Here's how the part is built. I have some questions about the finished solid (model axes, mm). A direction names the side the tool comes from. Round coordinates to 2 decimals unless told otherwise and drop trailing zeros. Loops run counter-clockwise (first coordinate to the right, second up) from the corner with the lowest first, then second, coordinate; pieces in that order, holes last. Notation, with made-up numbers: M 75,-8 L 130,-8 A8 ccw 130,1 Z; hole C 1,-13.75 d5. An arc over 180 degrees is marked long. Answer as CSV lines item,"result".
```python
from build123d import *

# Parameters (mm, degrees)
F0_W      = 45
F0_H      = 49
F1_DEPTH  = 80
F3_DEPTH  = 35
F4_W      = 72
F4_H      = 41
F5_DEPTH  = 55
F6_W      = 72
F6_H      = 23
F7_DEPTH  = 15
F9_W      = 80
F9_H      = 45
F9_R      = 8
F10_DEPTH = 14
F11_R     = 5
F13_DEPTH = 80


with BuildPart() as f1:
    # F0 (on Right) → F1 (new body)
    with BuildSketch(Plane.YZ):
        with Locations((22.5, -24.5)):
            Rectangle(F0_W, F0_H)
        Polygon((50, 86.6025403784), (0, 0), (45, 0), (95, 86.6025403784), align=None)
    extrude(amount=F1_DEPTH)

    # F2 (on face) → F3 (cut)
    with BuildSketch(Plane(origin=(0, 33.75, -19.4855715851), x_dir=(-1, 0, 0), z_dir=(0, 0.8660254038, -0.5))):
        Polygon((-76, 22.5), (-4, 22.5), (-4, 117.5), (-4, 122.5), (-76, 122.5), (-76, 117.5), align=None)
    extrude(amount=-F3_DEPTH, mode=Mode.SUBTRACT)

    # F4 (on face) → F5 (cut)
    with BuildSketch(Plane(origin=(0, 0, -49), x_dir=(1, 0, 0), z_dir=(0, 0, -1))):
        with Locations((40, -24.5)):
            Rectangle(F4_W, F4_H)
    extrude(amount=-F5_DEPTH, mode=Mode.SUBTRACT)

    # F6 (on face) → F7 (cut)
    with BuildSketch(Plane(origin=(0, 11.25, 19.4855715851), x_dir=(1, 0, 0), z_dir=(0, 0.5, 0.8660254038))):
        with Locations((40, 15.4711431703)):
            Rectangle(F6_W, F6_H)
    extrude(amount=-F7_DEPTH, mode=Mode.SUBTRACT)

    # F9 (on offset) → F10 (join)
    with BuildSketch(Plane.XY.offset(100)):
        with Locations((40, 72.5)):
            Rectangle(F9_W, F9_H)
        with Locations((40, 72.5)):
            Circle(F9_R, mode=Mode.SUBTRACT)
    extrude(amount=-F10_DEPTH)

    # F11
    f11_edges = [f1.edges().sort_by_distance(p)[0] for p in [
        (40, 95, 100),
    ]]
    fillet(f11_edges, radius=F11_R)

    # F12 (on face) → F13 (cut)
    with BuildSketch(Plane(origin=(0, 0, 0), x_dir=(0, -1, 0), z_dir=(-1, 0, 0))):
        Polygon((-30, -49), (-45, 0), (-45, -49), align=None)
    extrude(amount=-F13_DEPTH, mode=Mode.SUBTRACT)


solid = f1.part
```
1. I want a section at A-A, the plane x = 40. Please give me the cut outline in (y, z).
Evaluation:
outline,"M 0,-49 L 4,-49 L 4,6 L 8.05,6 L 54.24,86 L 64.5,86 L 64.5,100 L 50,100 L 50,86.6 L 0,0 Z; M 80.5,86 L 95,86 L 95,95 A5 ccw 90,100 L 80.5,100 Z"
2. Which directions (+Z, -Z, +X, -X, +Y, -Y) give clear straight access to the entire face, cutting with the end or side of a thin tool? Please do faces 1 (the flat face through (39, 4, -22)), 2 (the flat face through (39, 95, 91)), 3 (the flat face through (39, 50, 93)).
Evaluation:
face 1,"-Z, +Y"
face 2,"+Z, -Z, +X, -X, +Y"
face 3,"+Z, +X, -X, -Y"
3. If I drill on line 1 (X direction, y = 72, z = 91); line 2 (X direction, y = 38, z = 12); line 3 (Y direction, x = 40, z = 93), over which ranges is the centre line in solid material (lowest first)? Write a range as [from, to].
Evaluation:
line 1,"x = [0, 32.02], [47.98, 80]"
line 2,"x = [0, 4], [76, 80]"
line 3,"y = [50, 64.5], [80.5, 95]"
4. I want a section at C-C, the plane x = 54. Please give me the cut outline in (y, z), and give its area (3 significant figures).
Evaluation:
outline,"M 0,-49 L 4,-49 L 4,6 L 8.05,6 L 54.24,86 L 95,86 L 95,95 A5 ccw 90,100 L 50,100 L 50,86.6 L 0,0 Z"
area,"1,200 mm²"
5. I want a section at B-B, the plane y = 72.5. Please give me the cut outline in (x, z), and give its area (3 significant figures).
Evaluation:
outline,"M 0,47.63 L 4,47.63 L 4,86 L 32,86 L 32,100 L 0,100 Z; M 48,86 L 76,86 L 76,47.63 L 80,47.63 L 80,100 L 48,100 Z"
area,"1,200 mm²"
6. We'd pull the mould along Y, two halves only. Please class faces 4 (the flat face through (48, 75, 86)), 5 (the flat face through (39, 0, -25)), 6 (the cylindrical face through (38.959, 80.432, 93.098)): pulls with the +Y half, pulls with the -Y half, needs draft (parallel to the pull), parting line crosses it, or undercut.
Evaluation:
face 4,"needs draft"
face 5,"pulls with the -Y half"
face 6,"undercut"
7. For P1, Ø20.5, axis at x = 21.5, y = 75, coming from the -Z side; P2, Ø1.5, axis at x = 21.5, z = 77, coming from the +Y side; P3, Ø4.5, axis at x = 32, y = 7, coming from the -Z side, each with a flat end and sliding along its axis, tell me the tip position at first contact or that it passes through.
Evaluation:
P1,"stops at z = 86"
P2,"stops at y = 49.47"
P3,"stops at z = 6"
